Design review of the part built by this model. Coordinates are the model's own, in mm. A direction names the side the tool comes from. Coordinates: 2 decimals unless noted, no trailing zeros. Write each loop counter-clockwise with the first axis right and the second up, starting at its lowest first coordinate (ties: lowest second). Pieces come first, ordered by that corner, then holes. Notation, with made-up numbers: (60.5, -32.75) -> (81.5, -32.75) arc R12 ccw to (81.5, -15.75) -> close; hole circle Ø1 at (13.5, 52.5). An arc over 180 degrees is marked (long way). One line per question, with ' | ' between items. Start each with the question number.
Q1. Add section A-A on x = 29. State the section outline as (y, z) points.
Q2. Wall thickness on probe 1 along X at (y, z) = (-8, 15.5); probe 2 along Z at (x, y) = (16, -10.75); probe 3 along X at (y, z) = (-10, 65): over which ranges is each line inside the solid? List them lowest first.
Q3. Add section C-C on x = -50.5. State the section outline as (y, z) points, and give its area (3 significant figures).
Q4. Add section B-B on z = 4. State the section outline as (x, y) points.
Q5. Draft analysis for pull direction Z (two halves, no side actions). For faces 1 (the cylindrical face through (-41.273, -6.261, 16.188)), 2 (the flat face through (71, -6, -34.148)), 3 (the flat face through (-9.605, -6.261, 66.39)), 4 (the flat face through (101.346, -6, 23)), state which applies: pulls with the +Z half, pulls with the -Z half, needs draft (parallel to the pull), parting line crosses it, or undercut.
Q6. For P1, Ø1, axis at y = -9.5, z = 54.5, coming from the +X side; P2, Ø1.5, axis at y = -10, z = -22.5, coming from the +X side; P3, Ø4, axis at x = 89, y = -9, coming from the -Z side, all flat-tipped, find the tip position at first contact; note any pin that passes through.
Q7. For faces 5 (the flat face through (-1, -6, -21.702)), 6 (the flat face through (9.7, -6.26, 66.74)), 7 (the cylindrical face through (-32.825, -6.261, 75.679)), 8 (the flat face through (-75.946, -6, 9)), 9 (the flat face through (75.946, -6, 9)), list the 3-axis set-ups (+Z, -Z, +X, -X, +Y, -Y) from which the entire face can be reached by the end or side of a thin tool; tool diameter is ignored.
from build123d import *

# Parameters (mm, degrees)
F1_DEPTH     = 12.7
F2_T1_DEPTH  = 105.45546201
F2_T6_DEPTH  = 85.6153780659
F2_T11_DEPTH = 85.6153780659


# Not quite as in the source:
# - a fillet or chamfer that OpenCascade refuses, or shapes differently, is made with other operations: its cross-section is extruded or revolved along the edge and cut away or added


with BuildPart() as f1:
    # F0 (on Front) → F1 (new body)
    with BuildSketch(Plane.XZ):
        with BuildLine():
            Line((6.35, 54.2438933111), (-6.35, 54.2438933111))
            Line((-6.35, 54.2438933111), (-12.9517322031, 78.8818933111))
            Line((-12.9517322031, 78.8818933111), (-22.2531325433, 78.8818933111))
            ThreePointArc((-22.2531325433, 78.8818933111), (-32.9570059401, 75.5903702142), (-39.961976816, 66.8532417945))
            Line((-39.961976816, 66.8532417945), (-42.7458589128, 59.8318933111))
            ThreePointArc((-42.7458589128, 59.8318933111), (-53.7566077671, 45.7336602674), (-70.6412160864, 39.8254653493))
            Line((-70.6412160864, 39.8254653493), (-89.4780809568, 38.8634540506))
            ThreePointArc((-89.4780809568, 38.8634540506), (-97.258039529, 35.6807034492), (-101.346, 28.3358933111))
            Line((-101.346, 28.3358933111), (-101.346, 18.6838933111))
            Line((-101.346, 18.6838933111), (-75.946, 18.6838933111))
            Line((-75.946, 18.6838933111), (-75.946, -0.3661066889))
            Line((-75.946, -0.3661066889), (-101.346, -0.3661066889))
            Line((-101.346, -0.3661066889), (-101.346, -34.1481066889))
            Line((-101.346, -34.1481066889), (-45.212, -34.1481066889))
            Line((-45.212, -34.1481066889), (-42.0329745032, -21.7021066889))
            Line((-42.0329745032, -21.7021066889), (0, -21.7021066889))
            Line((0, -21.7021066889), (42.0329745032, -21.7021066889))
            Line((42.0329745032, -21.7021066889), (45.212, -34.1481066889))
            Line((45.212, -34.1481066889), (101.346, -34.1481066889))
            Line((101.346, -34.1481066889), (101.346, -0.3661066889))
            Line((101.346, -0.3661066889), (75.946, -0.3661066889))
            Line((75.946, -0.3661066889), (75.946, 18.6838933111))
            Line((75.946, 18.6838933111), (101.346, 18.6838933111))
            Line((101.346, 18.6838933111), (101.346, 28.3358933111))
            ThreePointArc((101.346, 28.3358933111), (97.258039529, 35.6807034492), (89.4780809568, 38.8634540506))
            Line((89.4780809568, 38.8634540506), (70.6412160864, 39.8254653493))
            ThreePointArc((70.6412160864, 39.8254653493), (53.7566077671, 45.7336602674), (42.7458589128, 59.8318933111))
            Line((42.7458589128, 59.8318933111), (39.961976816, 66.8532417945))
            ThreePointArc((39.961976816, 66.8532417945), (32.9570059401, 75.5903702142), (22.2531325433, 78.8818933111))
            Line((22.2531325433, 78.8818933111), (12.9517322031, 78.8818933111))
            Line((12.9517322031, 78.8818933111), (6.35, 54.2438933111))
        make_face()
        with BuildLine():
            ThreePointArc((-31.75, 6.8728933111), (-41.275, 16.3978933111), (-31.75, 25.9228933111))
            Line((-31.75, 25.9228933111), (31.75, 25.9228933111))
            ThreePointArc((31.75, 25.9228933111), (41.275, 16.3978933111), (31.75, 6.8728933111))
            Line((31.75, 6.8728933111), (-31.75, 6.8728933111))
        make_face(mode=Mode.SUBTRACT)
    extrude(amount=F1_DEPTH)

    # F2: chamfer of 18.034 on 4 edges, made by hand

    # F2_s2 → F2_t1 (cut)
    with BuildSketch(Plane.XZ.offset(-46.377731005)):
        Polygon((-101.346, -16.1141066889), (-83.312, -34.1481066889), (-101.346, -34.1481066889), align=None)
        Polygon((101.346, -16.1141066889), (83.312, -34.1481066889), (101.346, -34.1481066889), align=None)
    extrude(amount=F2_T1_DEPTH, mode=Mode.SUBTRACT)


with BuildPart() as f2_tool4:
    # F2_s5 → F2_t6 (new body)
    with BuildSketch(Plane.XZ.offset(-36.4576890329)):
        Polygon((-41.7456345338, -20.5771602982), (-59.218651116, -34.1481066889), (-45.212, -34.1481066889), align=None)
    extrude(amount=F2_T6_DEPTH)

    split(bisect_by=Plane.XY.offset(-21.7021066889), keep=Keep.BOTTOM)


with BuildPart() as f1_1:
    add(f1.part)

    # F2_t3: cut F2_tool4
    add(f2_tool4.part, mode=Mode.SUBTRACT)


with BuildPart() as f2_tool9:
    # F2_s10 → F2_t11 (new body)
    with BuildSketch(Plane.XZ.offset(-36.4576890329)):
        Polygon((59.218651116, -34.1481066889), (41.7456345338, -20.5771602982), (45.212, -34.1481066889), align=None)
    extrude(amount=F2_T11_DEPTH)

    split(bisect_by=Plane.XY.offset(-21.7021066889), keep=Keep.BOTTOM)


with BuildPart() as f1_2:
    add(f1_1.part)

    # F2_t8: cut F2_tool9
    add(f2_tool9.part, mode=Mode.SUBTRACT)


solid = f1_2.part
Output values:
1) outline: (-12.7, -21.7) -> (0, -21.7) -> (0, 6.87) -> (-12.7, 6.87) -> close; (-12.7, 25.92) -> (0, 25.92) -> (0, 77.65) -> (-12.7, 77.65) -> close
2) probe 1: x = -75.95 to -41.23, 41.23 to 75.95 | probe 2: z = -21.7 to 6.87, 25.92 to 78.88 | probe 3: x = -40.7 to -9.23, 9.23 to 40.7
3) outline: (-12.7, -27.38) -> (0, -27.38) -> (0, 48.41) -> (-12.7, 48.41) -> close | area: 963 mm2
4) outline: (-75.95, -12.7) -> (75.95, -12.7) -> (75.95, 0) -> (-75.95, 0) -> close
5) face 1: undercut | face 2: pulls with the -Z half | face 3: pulls with the +Z half | face 4: needs draft
6) P1: stops at x = 45.79 | P2: stops at x = 95.71 | P3: stops at z = -30.46
7) face 5: -Z, +Y, -Y | face 6: +Z, +Y, -Y | face 7: +Z, -X, +Y, -Y | face 8: -X, +Y, -Y | face 9: +X, +Y, -Y
